Autodesk Fusion 360 part; units mm, degrees
sketch "Sketch1" plane through (0, 0, 0) normal (0, 0, 1) x (1, 0, 0)
  line L0 (-29, 18) -> (29, 18)
  line L1 (29, 18) -> (29, -18)
  line L2 (29, -18) -> (-29, -18)
  line L3 (-29, -18) -> (-29, 18)
  line L4 (-29, 18) -> (29, -18) construction
  line L5 (29, 18) -> (-29, -18) construction
  line L6 (29, 8.6) -> (-29, 8.6) construction
  line L7 (-29, -18) -> (-29, -26)
  line L8 (-29, -26) -> (29, -26)
  line L9 (29, -26) -> (29, -18)
  line L10 (29, -26) -> (29, -29)
  line L11 (29, -29) -> (-29, -29)
  line L12 (-29, -29) -> (-29, -26)
  line L13 (-29, 5.6) -> (-20.5, 5.6)
  line L14 (-20.5, 5.6) -> (-20.5, 8.6)
  line L15 (-20.5, 8.6) -> (-29, 8.6)
  line L16 (-20.5, 5.6) -> (-20.5, 0.6)
  line L17 (-20.5, 0.6) -> (-19, 0.6)
  line L18 (-19, 0.6) -> (-19, 8.6)
  line L19 (0, -29) -> (0, 18) construction
  line L20 (20.5, 8.6) -> (29, 8.6)
  line L21 (20.5, 5.6) -> (20.5, 8.6)
  line L22 (29, 5.6) -> (20.5, 5.6)
  line L23 (20.5, 5.6) -> (20.5, 0.6)
  line L24 (20.5, 0.6) -> (19, 0.6)
  line L25 (19, 0.6) -> (19, 8.6)
  circle A0 centre (0, 0) radius 4
  circle A1 centre (0, 0) radius 7 construction
  circle A2 centre (0, 7) radius 1.25
  circle A3 centre (-7, 0) radius 1.25
  circle A4 centre (0, -7) radius 1.25
  circle A5 centre (7, 0) radius 1.25
  line L26 (-19, 8.6) -> (-20.5, 8.6)
  line L27 (19, 8.6) -> (20.5, 8.6)
  line L28 (-19, 8.6) -> (-19, 18)
  line L29 (19, 8.6) -> (19, 18)
  line L30 (-21, -14) -> (-15, -14)
  line L31 (-15, -14) -> (-15, -16)
  line L32 (-15, -16) -> (-21, -16)
  line L33 (-21, -16) -> (-21, -14)
  line L34 (15, -14) -> (15, -16)
  line L35 (21, -16) -> (21, -14)
  line L36 (15, -16) -> (21, -16)
  line L37 (21, -14) -> (15, -14)
  line L38 (0, -7) -> (29, -7) construction
  circle A6 centre (0, -14) radius 4
  circle A7 centre (0, -21) radius 1.25
  circle A8 centre (7, -14) radius 1.25
  circle A9 centre (-7, -14) radius 1.25
  dimension "d4" = 36
  dimension "d5" = 58
  dimension "d9" = 26.6
  dimension "d11" = 8
  dimension "d12" = 8
  dimension "d13" = 3
  dimension "d14" = 3
  dimension "d16" = 8.5
  dimension "d17" = 3
  dimension "d18" = 1.5
  dimension "d19" = 8
  dimension "d22" = 8
  dimension "d23" = 14
  dimension "d24" = 2.5
  dimension "d26" = 360
  dimension "d56" = 2
  dimension "d57" = 6
  dimension "d58" = 8
  dimension "d59" = 2
extrude "Extrude3" add sketch "Sketch1" against normal blind 3 contours L0 L1 L2 L3 L13 L16 L17 L18 L22 L23 L24 L25 L28 L29 | L3 L13 L14 L15 | L2 L7 L8 L9 | L1 L20 L21 L22 | L8 L10 L11 L12 | L30 L31 L32 L33 | L34 L35 L36 L37
extrude "Extrude4" add sketch "Sketch1" along normal blind 25 contours L3 L13 L14 L15 | L1 L20 L21 L22 | L8 L10 L11 L12
fillet "Fillet1" radius 2.5 6 edges at (29, -27.5, 25) (-29, -27.5, 25) (29, 7.1, 25) (-29, 7.1, 25) (-20.5, 7.1, 25) (20.5, 7.1, 25)
fillet "Fillet2" radius 5 2 edges at (19, 18, -1.5) (-19, 18, -1.5)
fillet "Fillet3" radius 2 6 edges at (0, -26, 0) (0, -29, -3) (24.75, 5.6, 0) (24.75, 8.6, -3) (-24.75, 8.6, -3) (-24.75, 5.6, 0)
fillet "Fillet3" radius 1 6 edges at (-19, 6.8, -3) (-17.5355, 16.5355, -3) (0, 18, -3) (17.5355, 16.5355, -3) (19, 10.8, -3) (19, 4.6, -3)
sketch "Sketch3" plane through (0, 5.6, 0) normal (0, -1, 0) x (1, 0, 0)
  line L0 (-29, 2) -> (-20.5, 2)
  line L1 (-20.5, 2) -> (-20.5, 22.5)
  arc A0 (-20.5, 22.5) -> (-23, 25) centre (-23, 22.5) ccw
  line L2 (-23, 25) -> (-26.5, 25)
  arc A1 (-26.5, 25) -> (-29, 22.5) centre (-26.5, 22.5) ccw
  line L3 (-29, 22.5) -> (-29, 2)
  line L4 (0, 0) -> (0, 25) construction
  line L5 (0, 0) -> (-24.25, 0) construction
  line L6 (-24.25, 0) -> (-24.25, 25) construction
  line L7 (-24.25, 12.5) -> (0, 12.5) construction
  circle A2 centre (-24.25, 8) radius 2
  circle A3 centre (-24.25, 18) radius 2
  line L8 (-7.25, 14.5877) -> (-10, 16.1754)
  line L9 (-10, 16.1754) -> (-12.75, 14.5877)
  line L10 (-12.75, 14.5877) -> (-12.75, 11.4123)
  line L11 (-12.75, 11.4123) -> (-10, 9.8246)
  line L12 (-10, 9.8246) -> (-7.25, 11.4123)
  line L13 (-7.25, 11.4123) -> (-7.25, 14.5877)
  circle A4 centre (24.25, 18) radius 2
  circle A5 centre (24.25, 8) radius 2
  line L14 (12.75, 11.4123) -> (10, 9.8246)
  line L15 (12.75, 14.5877) -> (12.75, 11.4123)
  line L16 (10, 16.1754) -> (12.75, 14.5877)
  line L17 (7.25, 14.5877) -> (10, 16.1754)
  line L18 (7.25, 11.4123) -> (7.25, 14.5877)
  line L19 (10, 9.8246) -> (7.25, 11.4123)
  point P0 (-10, 13)
  dimension "d49" = 25
  dimension "d50" = 24.25
  dimension "d51" = 25
  dimension "d52" = 4
  dimension "d53" = 4.5
  dimension "d54" = 10
  dimension "d55" = 4
  dimension "d64" = 2.75
  dimension "d65" = 0.5
  dimension "d66" = 14.25
extrude "Extrude5" add sketch "Sketch1" along normal blind 3 contours L30 L31 L32 L33 | L34 L35 L36 L37
fillet "Fillet4" radius 0.5 8 edges at (18, -14, 0) (21, -15, 0) (18, -16, 0) (15, -15, 0) (-15, -15, 0) (-18, -14, 0) (-21, -15, 0) (-18, -16, 0)
extrude "Extrude6" cut sketch "Sketch3" against normal through all contours A2 | A3 | A4 | A5
extrude "Extrude7" cut sketch "Sketch3" along normal blind 42 contours L8 L9 L10 L11 L12 L13 | L14 L15 L16 L17 L18 L19
equation "thickness = 3 mm"
equation "base_width = 36 mm"
equation "base_length = 58 mm"
equation "d4 = base_width"
equation "d5 = base_length"
equation "d9 = servoHolder_height"
equation "servo_clearence = 8 mm"
equation "d11 = servo_clearence"
equation "d12 = servo_clearence"
equation "d13 = thickness"
equation "d14 = thickness"
equation "servoHolder_height = 26.6 mm"
equation "d17 = thickness"
equation "main_hole = 8 mm"
equation "titner_hole = 2.5 mm"
equation "d22 = main_hole"
equation "d24 = titner_hole"
equation "base_height = 25 mm"
equation "d34 = base_height"
equation "d50 = ( 48.5 / 2 ) * 1 mm"
equation "d64 = ( 5.5 / 2 ) * 1 mm"
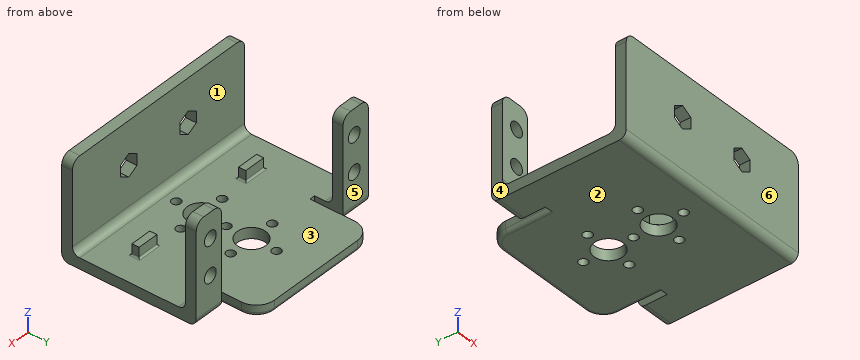
Could you check a few things on this model? Use its own coordinates, in mm. Face numbers are marked on the shaded views. A direction names the side the tool comes from. Give positions to 0.01 mm unless a question says otherwise; leave off trailing zeros. Write each loop counter-clockwise with the first axis right and the second up, starting at its lowest first coordinate (ties: lowest second). Pieces come first, ordered by that corner, then holes. Notation, with made-up numbers: (4.25, 64.25) -> (26.25, 64.25) arc R36 ccw to (26.25, 98.25) -> close; hole circle Ø5 at (-27, 45). An arc over 180 degrees is marked (long way). Answer as CSV lines item,"result". Start each with the question number.
(1) I'm going to push flat-ended pins straight in: pin 1 Ø4 at (y, z) = (3.5, 15.5) entering from +X; pin 2 Ø3 at (x, y) = (7, 0) entering from +Z; pin 3 Ø1 at (x, y) = (17.5, -14.5) entering from +Z; pin 4 Ø4 at (x, z) = (22.5, 10) entering from +Y. Where does each tip first touch, or does it pass through?
(2) Please list where these lines run through material, in increasing order: line 1 (X direction, y = 8.5, z = 7.75); line 2 (Y direction, x = 7, z = -1.2); line 3 (Y direction, x = 0, z = -1.25).
(3) If we section it at C-C, the plane y = -7: Write out the boundary of the cut face in (x, z), and give its area (4 significant figures).
(4) If we section it at D-D, the plane z = 17.25: Write out the boundary of the cut face in (x, y).
(5) If we section it at A-A, the plane z = 4.5: Write out the boundary of the cut face in (x, y), and give its area (3 significant figures).
(6) If we mould it in two halves opening along Y, with no side actions, what happens to the marked faces 3, 4, 5 and 6? For each: +Y half, -Y half, draft (parallel to the pull), parting line (faces both ways), or undercut.
(7) If we section it at B-B, the plane x = 0: Give the number of separate pieces and of enclosed holes in the cut face, and give its area (3 significant figures).
(8) Which directions (+Z, -Z, +X, -X, +Y, -Y) give clear straight access to the entire face, cutting with the end or side of a thin tool? Please do the marked faces 1 and 2.
Answer list:
1,pin 1,"through"
1,pin 2,"z = 0"
1,pin 3,"z = 3"
1,pin 4,"y = 8.6"
2,line 1,"-29 to -26.23, -22.27 to -20.5, 20.5 to 22.27, 26.23 to 29"
2,line 2,"-28.99 to -15.25, -12.75 to -1.25, 1.25 to 18"
2,line 3,"-28.98 to -22.25, -19.75 to -18, -10 to -8.25, -5.75 to -4, 4 to 5.75, 8.25 to 18"
3,outline,"(-29, -3) -> (-1.25, -3) -> (-1.25, 0) -> (-29, 0) -> close; (1.25, -3) -> (29, -3) -> (29, 0) -> (1.25, 0) -> close"
3,area,"166.5 mm^2"
4,outline,"(-29, -29) -> (29, -29) -> (29, -26) -> (-29, -26) -> close; (-29, 5.6) -> (-26.1, 5.6) -> (-26.1, 8.6) -> (-29, 8.6) -> close; (-22.4, 5.6) -> (-20.5, 5.6) -> (-20.5, 8.6) -> (-22.4, 8.6) -> close; (20.5, 5.6) -> (22.4, 5.6) -> (22.4, 8.6) -> (20.5, 8.6) -> close; (26.1, 5.6) -> (29, 5.6) -> (29, 8.6) -> (26.1, 8.6) -> close"
5,outline,"(-29, -29) -> (29, -29) -> (29, -26) -> (-29, -26) -> close; (-29, 5.6) -> (-20.5, 5.6) -> (-20.5, 8.6) -> (-29, 8.6) -> close; (20.5, 5.6) -> (29, 5.6) -> (29, 8.6) -> (20.5, 8.6) -> close"
5,area,"225 mm^2"
6,face 3,"undercut"
6,face 4,"draft"
6,face 5,"+Y half"
6,face 6,"-Y half"
7,separate pieces,"6"
7,enclosed holes,"0"
7,area,"145 mm^2"
8,face 1,"+Z, +X, -X"
8,face 2,"-Z, +X, -X, +Y, -Y"
